The drawing under review shows one solid part. Ordinate dimensions are in mm from its lowest x, y, z. Round coordinates to 2 decimals unless told otherwise and drop trailing zeros. Write each loop counter-clockwise with the first axis right and the second up, starting at its lowest first coordinate (ties: lowest second). Pieces come first, ordered by that corner, then holes. Notation, with made-up numbers: (78.5, 80.25) -> (115.5, 80.25) arc R32 cw to (115.5, 108.25) -> close; hole circle Ø2 at (-39.75, 72.5). An arc over 180 degrees is marked (long way). Use CSV: the item, a comma, the result in double quotes. Start each with the question number.
1) Take a section at C-C, the plane y = 5.75. Give the boundary of the cut face in (x, z).
2) Wall thickness on probe 1 along X at (y, z) = (4.25, 108); probe 2 along Z at (x, y) = (39, 1.5); probe 3 along X at (y, z) = (1.25, 32.5): over which ranges is each line inside the solid? List them lowest first. Write a range as [from, to].
3) Take a section at B-B, the plane z = 132.5. Give the boundary of the cut face in (x, y), then the cut area to 3 significant figures.
4) Take a section at A-A, the plane x = 86. Give the boundary of the cut face in (y, z), then the cut area to 3 significant figures.
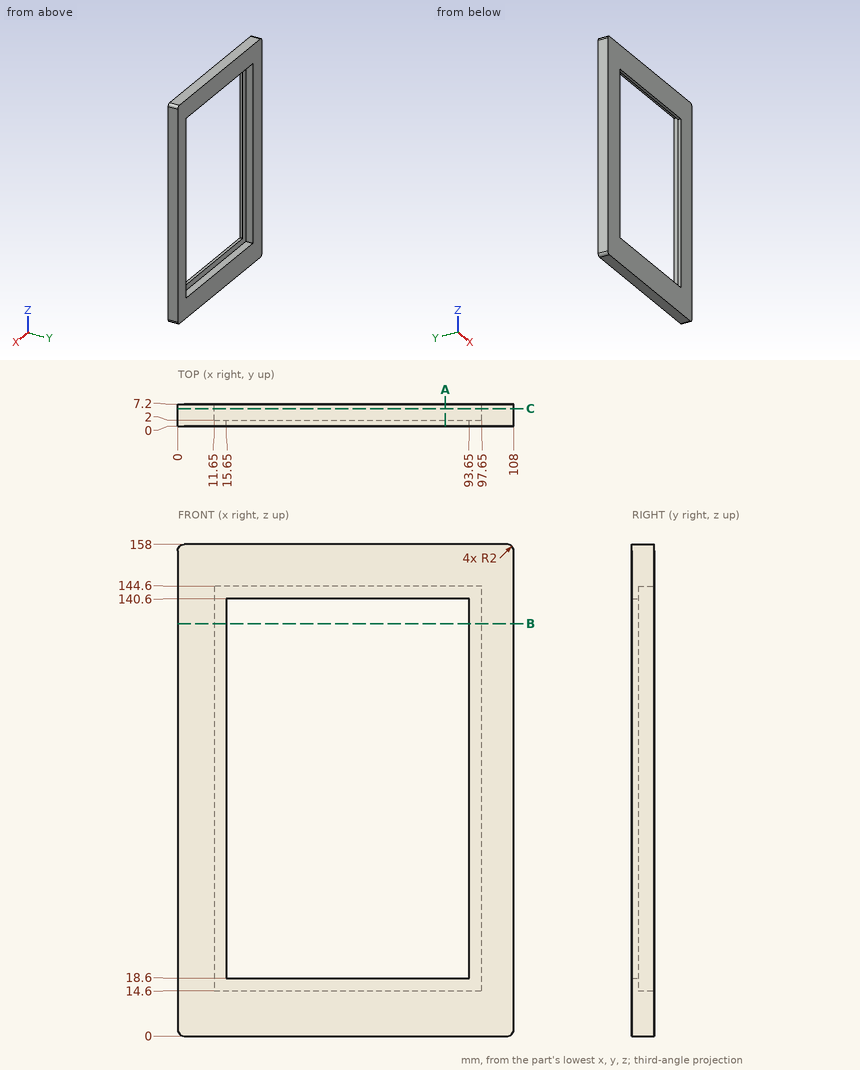
Values found:
1,outline,"(0, 2) arc R2 ccw to (2, 0) -> (106, 0) arc R2 ccw to (108, 2) -> (108, 156) arc R2 ccw to (106, 158) -> (2, 158) arc R2 ccw to (0, 156) -> close; hole (11.65, 14.6) -> (97.65, 14.6) -> (97.65, 144.6) -> (11.65, 144.6) -> close"
2,probe 1,"[0, 11.65], [97.65, 108]"
2,probe 2,"[0, 18.6], [140.6, 158]"
2,probe 3,"[0, 15.65], [93.65, 108]"
3,outline,"(0, 0) -> (15.65, 0) -> (15.65, 2) -> (11.65, 2) -> (11.65, 7.2) -> (0, 7.2) -> close; (93.65, 0) -> (108, 0) -> (108, 7.2) -> (97.65, 7.2) -> (97.65, 2) -> (93.65, 2) -> close"
3,area,"174 mm²"
4,outline,"(0, 0) -> (7.2, 0) -> (7.2, 14.6) -> (2, 14.6) -> (2, 18.6) -> (0, 18.6) -> close; (0, 140.6) -> (2, 140.6) -> (2, 144.6) -> (7.2, 144.6) -> (7.2, 158) -> (0, 158) -> close"
4,area,"218 mm²"
